```python
from build123d import *

# Parameters (mm, degrees)
SKETCH2_W           = 47.498
SKETCH2_H           = 37.846
BOSS_EXTRUDE1_DEPTH = 3.175
SKETCH4_W           = 47.498
SKETCH4_H           = 37.846
SKETCH4_W_2         = 41.148
SKETCH4_H_2         = 31.496
BOSS_EXTRUDE2_DEPTH = 12.7
SKETCH5_R           = 4.7625
SKETCH5_R_2         = 6.35
BOSS_EXTRUDE3_DEPTH = 6.35
SKETCH6_R           = 4.7625
SKETCH6_R_2         = 3.175
CUT_EXTRUDE1_DEPTH  = 5.08
SKETCH7_R           = 1.524
SKETCH7_R_2         = 3.937
CUT_EXTRUDE2_DEPTH  = 43.987201933


with BuildPart() as part:
    # Sketch2 → Boss-Extrude1 (new body)
    with BuildSketch(Plane.XY):
        with Locations((12.7, 0)):
            Rectangle(SKETCH2_W, SKETCH2_H)
    extrude(amount=BOSS_EXTRUDE1_DEPTH)

    # Sketch4 → Boss-Extrude2 (add)
    with BuildSketch(Plane.XY.offset(3.175)):
        with Locations((12.7, 0)):
            Rectangle(SKETCH4_W, SKETCH4_H)
        with Locations((12.7, 0)):
            Rectangle(SKETCH4_W_2, SKETCH4_H_2, mode=Mode.SUBTRACT)
    extrude(amount=BOSS_EXTRUDE2_DEPTH)

    # Sketch5 → Boss-Extrude3 (add)
    with BuildSketch(Plane(origin=(0, 0, 0), x_dir=(-1, 0, 0), z_dir=(0, 0, -1))):
        Circle(SKETCH5_R)
        with Locations((-17.526, 0)):
            Circle(SKETCH5_R_2)
    extrude(amount=-BOSS_EXTRUDE3_DEPTH)

    # Sketch6 → Cut-Extrude1 (cut)
    with BuildSketch(Plane.XY.offset(6.35)):
        with Locations((17.526, 0)):
            Circle(SKETCH6_R)
        Circle(SKETCH6_R_2)
    extrude(amount=-CUT_EXTRUDE1_DEPTH, mode=Mode.SUBTRACT)

    # Sketch7 → Cut-Extrude2 (cut, through all)
    with BuildSketch(Plane.XY.offset(3.175)):
        Circle(SKETCH7_R)
        with Locations((17.526, 0)):
            Circle(SKETCH7_R_2)
    extrude(amount=-CUT_EXTRUDE2_DEPTH, mode=Mode.SUBTRACT)


solid = part.part
```
Here's how the part is built. I have some questions about the finished solid (model axes, mm). A direction names the side the tool comes from. Round coordinates to 2 decimals unless told otherwise and drop trailing zeros. Write each loop counter-clockwise with the first axis right and the second up, starting at its lowest first coordinate (ties: lowest second). Pieces come first, ordered by that corner, then holes.
Q1. If we section it at A-A on y = 0: Give the number of separate pieces and of enclosed holes in the cut face, plus the area to 4 significant figures.
Q2. Will these pins go through, and if not, where does the flat tip stop? P1, Ø3, axis at x = -1, y = 0, coming from the -Z side; P2, Ø3.5, axis at x = 0, y = 0, coming from the +Z side; P3, Ø15, axis at x = 17.526, y = 0, coming from the +Z side; P4, Ø7, axis at x = 17.526, y = 0, coming from the +Z side.
Q3. If we section it at B-B on z = 14.5: Write out the boundary of the cut face in (x, y), plus the area to 3 significant figures.
Q4. If we section it at D-D on y = 13: Write out the boundary of the cut face in (x, z) (3 decimals), plus the area to 3 significant figures.
Q5. Please list where these lines run through material, in increasing order: probe 1 along Y at (x, z) = (0, 5.15) (1 decimal); probe 2 along Y at (x, z) = (-6, 15.25); probe 3 along X at (y, z) = (15, 10.5).
Q6. If we mould it in two halves opening along Y, with no side actions, what happens to faces 3 (the flat face through (12, -17, 15.875)), 4 (the flat face through (12, 18.923, 8)), 5 (the flat face through (-0.8, 1.5, 1.27))? For each: +Y half, -Y half, draft (parallel to the pull), parting line (faces both ways), or undercut.
Q7. Which directions (+Z, -Z, +X, -X, +Y, -Y) give clear straight access to the entire face, cutting with the end or side of a thin tool? Please do faces 1 (the flat face through (33.274, 0, 9)), 2 (the flat face through (36.449, 0, 8)).
Answer below:
1. separate pieces: 3
1. enclosed holes: 0
1. area: 207.5 mm2
2. P1: stops at z = 0
2. P2: stops at z = 1.27
2. P3: stops at z = 6.35
2. P4: passes through
3. outline: (-11.05, -18.92) - (36.45, -18.92) - (36.45, 18.92) - (-11.05, 18.92) - close; hole (-7.87, -15.75) - (33.27, -15.75) - (33.27, 15.75) - (-7.87, 15.75) - close
3. area: 502 mm2
4. outline: (-11.049, 0) - (36.449, 0) - (36.449, 15.875) - (33.274, 15.875) - (33.274, 3.175) - (-7.874, 3.175) - (-7.874, 15.875) - (-11.049, 15.875) - close
4. area: 231 mm2
5. probe 1: y = -18.9 to -15.7, -4.8 to -3.2, 3.2 to 4.8, 15.7 to 18.9
5. probe 2: y = -18.92 to -15.75, 15.75 to 18.92
5. probe 3: x = -11.05 to -7.87, 33.27 to 36.45
6. face 3: draft
6. face 4: +Y half
6. face 5: undercut
7. face 1: +Z
7. face 2: +Z, -Z, +X, +Y, -Y
